Work out the finished part from the listing and answer in its coordinate system (mm). A direction names the side the tool comes from. Give positions to 0.01 mm unless a question says otherwise; leave off trailing zeros. Loops run counter-clockwise (first coordinate to the right, second up) from the corner with the lowest first, then second, coordinate; pieces in that order, holes last. Notation, with made-up numbers: (-3.75, 81) - (0.25, 81) arc R17 ccw to (0.25, 94) - close; hole circle Ø8 at (64, 7.5). An arc over 180 degrees is marked (long way). Use CSV: the item, a comma, the result in double quotes.
from build123d import *

# Parameters (mm, degrees)
BOSS_EXTRUDE1_DEPTH          = 54.00000000000001
CUT_EXTRUDE1_REACH           = 79.096
SKETCH4_W                    = 49.00000000000001
SKETCH4_H                    = 9.930000000000003
CUT_EXTRUDE2_DEPTH           = 9.930000000000001
CUT_EXTRUDE3_DEPTH           = 9.930000000000001
CUT_EXTRUDE4_REACH           = 79.096
CUT_EXTRUDE5_DEPTH           = 3.5
CUT_EXTRUDE6_DEPTH           = 3.5
CUT_EXTRUDE7_DEPTH           = 3.5
CUT_EXTRUDE8_DEPTH           = 3.5
DRAFT1_ANGLE                 = 0.01722183664478431
F_5_0_5_DIAMETER_HOLE1_D     = 5
F_5_0_5_DIAMETER_HOLE1_DEPTH = 29.6
F_5_0_5_DIAMETER_HOLE2_D     = 5
F_5_0_5_DIAMETER_HOLE2_DEPTH = 26.5
FILLET1_R                    = 2
FILLET2_R                    = 5
FILLET3_R                    = 0.4999999999999998
FILLET5_R                    = 2.9999999999999996
BOSS_EXTRUDE2_DEPTH          = 21
FILLET4_R                    = 0.9999999999999991


with BuildPart() as part:
    # Sketch1 → Boss-Extrude1 (new body)
    with BuildSketch(Plane(origin=(0, 0, 0), x_dir=(-1, 0, 0), z_dir=(0, 0, -1))):
        Polygon((-28.5, 28.5), (-28.5, -28.51414849795304), (28.5, -28.49701556553382), (28.5, 28.5), align=None)
    extrude(amount=-BOSS_EXTRUDE1_DEPTH)

    # Cut-Extrude1: up to this plane
    cut_extrude1_end = Plane(origin=(28.5, -28.51414849795304, 54.00000000000001), z_dir=(-0.0003005777481625158, -0.9999999548265077, 0))
    # Sketch3 → Cut-Extrude1 (cut, up to the surface)
    with BuildSketch(Plane(origin=(0, -18.57, 0), x_dir=(1, 0, 0), z_dir=(0, 1, 0)), mode=Mode.PRIVATE) as cut_extrude1_sk1:
        Polygon((28.499999999999996, -5.000000000000003), (18.57, -5.000000000000004), (18.570000000000004, -54), (28.499999999999996, -53.99999999999999), align=None)
    cut_extrude1_tool1 = split(extrude(cut_extrude1_sk1.sketch, amount=-CUT_EXTRUDE1_REACH, mode=Mode.PRIVATE), bisect_by=cut_extrude1_end, keep=Keep.BOTH, mode=Mode.PRIVATE)
    add(cut_extrude1_tool1.solids().sort_by_distance((23.535, -18.57, 29.5))[0], mode=Mode.SUBTRACT)

    # Sketch4 → Cut-Extrude2 (cut)
    with BuildSketch(Plane(origin=(28.5, 0, 0), x_dir=(0, 0, -1), z_dir=(1, 0, 0))):
        with Locations((-29.500000000000004, 23.535000000000004)):
            Rectangle(SKETCH4_W, SKETCH4_H)
    extrude(amount=-CUT_EXTRUDE2_DEPTH, mode=Mode.SUBTRACT)

    # Sketch5 → Cut-Extrude3 (cut)
    with BuildSketch(Plane(origin=(0, 28.5, 0), x_dir=(-1, 0, 0), z_dir=(0, 1, 0))):
        Polygon((18.570000000000004, 5.000000000000003), (28.499999999999996, 5.000000000000003), (28.5, 54), (18.57, 54), align=None)
    extrude(amount=-CUT_EXTRUDE3_DEPTH, mode=Mode.SUBTRACT)

    # Cut-Extrude4: up to this plane
    cut_extrude4_end = Plane(origin=(28.5, -28.51414849795304, 54.00000000000001), z_dir=(-0.0003005777481625158, -0.9999999548265077, 0))
    # Sketch7 → Cut-Extrude4 (cut, up to the surface)
    with BuildSketch(Plane(origin=(0, -18.57, 0), x_dir=(1, 0, 0), z_dir=(0, 1, 0)), mode=Mode.PRIVATE) as cut_extrude4_sk1:
        Polygon((-18.569999999999997, -5.000000000000004), (-28.499999999999996, -5.000000000000003), (-28.5, -54), (-18.569999999999997, -53.99999999999999), align=None)
    cut_extrude4_tool1 = split(extrude(cut_extrude4_sk1.sketch, amount=-CUT_EXTRUDE4_REACH, mode=Mode.PRIVATE), bisect_by=cut_extrude4_end, keep=Keep.BOTH, mode=Mode.PRIVATE)
    add(cut_extrude4_tool1.solids().sort_by_distance((-23.535, -18.57, 29.5))[0], mode=Mode.SUBTRACT)

    # Sketch8 → Cut-Extrude5 (cut)
    with BuildSketch(Plane(origin=(0, 0, 0), x_dir=(-1, 0, 0), z_dir=(0, 0, -1))):
        with BuildLine():
            Line((18.5710070868336, -28.5), (18.569999848669397, -25.148993064543653))
            ThreePointArc((18.569999848669397, -25.148993064543653), (15.21959273974545, -21.800000024754763), (11.870000005525402, -25.149807585039706))
            Line((11.870000005525402, -25.149807585039706), (11.869807463820973, -28.502014231583665))
            Line((11.869807463820973, -28.502014231583665), (18.5710070868336, -28.5))
        make_face()
    extrude(amount=-CUT_EXTRUDE5_DEPTH, mode=Mode.SUBTRACT)

    # Sketch9 → Cut-Extrude6 (cut)
    with BuildSketch(Plane(origin=(0, 0, 0), x_dir=(-1, 0, 0), z_dir=(0, 0, -1))):
        with BuildLine():
            Line((-18.57, 28.5), (-18.57, 25.15))
            ThreePointArc((-18.57, 25.15), (-15.22, 21.799999999999997), (-11.87, 25.15))
            Line((-11.87, 25.15), (-11.87, 28.5))
            Line((-11.87, 28.5), (-18.57, 28.5))
        make_face()
    extrude(amount=-CUT_EXTRUDE6_DEPTH, mode=Mode.SUBTRACT)

    # Sketch10 → Cut-Extrude7 (cut)
    with BuildSketch(Plane(origin=(0, 0, 0), x_dir=(-1, 0, 0), z_dir=(0, 0, -1))):
        with BuildLine():
            Line((-25.15, -11.870000000000003), (-28.5, -11.87))
            Line((-28.5, -11.87), (-28.5, -18.57))
            Line((-28.5, -18.57), (-25.15, -18.57))
            ThreePointArc((-25.15, -18.57), (-21.799999999999997, -15.22), (-25.15, -11.870000000000003))
        make_face()
    extrude(amount=-CUT_EXTRUDE7_DEPTH, mode=Mode.SUBTRACT)

    # Sketch11 → Cut-Extrude8 (cut)
    with BuildSketch(Plane(origin=(0, 0, 0), x_dir=(-1, 0, 0), z_dir=(0, 0, -1))):
        with BuildLine():
            Line((28.5, 18.57), (25.15, 18.57))
            ThreePointArc((25.15, 18.57), (21.799999999999997, 15.22), (25.15, 11.869999999999992))
            Line((25.15, 11.869999999999992), (28.5, 11.87))
            Line((28.5, 11.87), (28.5, 18.57))
        make_face()
    extrude(amount=-CUT_EXTRUDE8_DEPTH, mode=Mode.SUBTRACT)

    # Draft1
    draft1_faces = [part.faces().sort_by_distance(p)[0] for p in [
        (0.17151026292326854, -28.505633583914378, 26.11567870035269),
    ]]
    draft(draft1_faces, Plane(origin=(-18.5710070868336, -28.5, 3.5), x_dir=(0.00030057774815282144, 0.9999999548265077, 0), z_dir=(0.9999999548265077, -0.00030057774815282144, 0)), DRAFT1_ANGLE)

    # Sketch12 → Revolve1 (revolve)
    with BuildSketch(Plane(origin=(0, 0, 0), x_dir=(1, 0, 0), z_dir=(0, 1, 0))):
        Polygon((3.2500000000000004, 24.6), (0, 24.6), (0, 0), (19.05, 0), (19.05, 1.6), (3.2500000000000004, 1.6000000000000008), align=None)
    revolve(axis=Axis((0, 0, -24.6), (0, 0, 1)))

    # Ø5.0 (5) Diameter Hole1
    with Locations(Plane.XY.offset(5.000000000000008)):
        with Locations((23.57, -23.57), (23.57, 23.57), (-23.57, 23.57), (-23.57, -23.57)):
            Hole(F_5_0_5_DIAMETER_HOLE1_D / 2, depth=F_5_0_5_DIAMETER_HOLE1_DEPTH)

    # Ø5.0 (5) Diameter Hole2
    with Locations(Plane(origin=(0, 0, 3.5), x_dir=(-1, 0, 0), z_dir=(0, 0, -1))):
        with Locations((15.22, -25.15), (-25.15, -15.22), (-15.22, 25.15), (25.15, 15.22)):
            Hole(F_5_0_5_DIAMETER_HOLE2_D / 2, depth=F_5_0_5_DIAMETER_HOLE2_DEPTH)

    # Fillet1
    fillet1_edges = [part.edges().sort_by_distance(p)[0] for p in [
        (28.499999999999996, -18.57, 29.499999999999996),
        (18.570000000000004, -28.49999999999951, 29.50000000000001),
        (18.57, 28.5, 29.500000000000004),
        (28.5, 18.57, 29.5),
        (-28.499999999999996, 18.57, 29.500000000000004),
        (-18.57, 28.5, 29.5),
        (-28.499999999999996, -18.57, 29.500000000000004),
        (-18.57, -28.5, 29.500000000000007),
    ]]
    fillet(fillet1_edges, radius=FILLET1_R)

    # Fillet2
    fillet2_edges = [part.edges().sort_by_distance(p)[0] for p in [
        (18.57, -18.57, 29.5),
        (18.57, 18.57, 29.5),
        (-18.57, 18.57, 29.5),
        (-18.569999999999997, -18.57, 29.5),
    ]]
    fillet(fillet2_edges, radius=FILLET2_R)

    # Fillet3
    fillet3_edges = [part.edges().sort_by_distance(p)[0] for p in [
        (-3.2500000000000004, 4e-16, -24.6),
    ]]
    fillet(fillet3_edges, radius=FILLET3_R)

    # Fillet5
    fillet5_edges = [part.edges().sort_by_distance(p)[0] for p in [
        (28.5, -28.499999999999375, 2.5000000000000013),
        (28.5, 28.5, 2.5000000000000013),
        (-28.5, 28.5, 2.5000000000000013),
        (-28.5, -28.500000000000135, 2.5000000000000013),
    ]]
    fillet(fillet5_edges, radius=FILLET5_R)

    # Sketch17 → Boss-Extrude2 (add)
    with BuildSketch(Plane.XY.offset(54.00000000000001)):
        with BuildLine():
            Line((-16.570000000000007, 28.5), (16.569999999999983, 28.5))
            ThreePointArc((16.569999999999983, 28.5), (17.98421356237308, 27.914213562373096), (18.57, 26.500000000000004))
            Line((18.57, 26.500000000000004), (18.57, 23.57))
            ThreePointArc((18.57, 23.57), (20.034466094067263, 20.034466094067263), (23.57, 18.57))
            Line((23.57, 18.57), (26.499999999999996, 18.57))
            ThreePointArc((26.499999999999996, 18.57), (27.914213562373096, 17.984213562373093), (28.5, 16.569999999999993))
            Line((28.5, 16.569999999999993), (28.500000000000004, -16.569999999999997))
            ThreePointArc((28.500000000000004, -16.569999999999997), (27.9142135623731, -17.984213562373093), (26.500000000000004, -18.57))
            Line((26.500000000000004, -18.57), (23.569999999999986, -18.57))
            ThreePointArc((23.569999999999986, -18.57), (20.034466094067255, -20.034466094067263), (18.57, -23.57))
            Line((18.57, -23.57), (18.570000000000004, -26.499999999999538))
            ThreePointArc((18.570000000000004, -26.499999999999538), (17.98421356237311, -27.914213562372627), (16.57000000000003, -28.499999999999535))
            Line((16.57000000000003, -28.499999999999535), (-16.56999999999997, -28.49999999999997))
            ThreePointArc((-16.56999999999997, -28.49999999999997), (-17.98421356237307, -27.91421356237308), (-18.569999999999993, -26.49999999999999))
            Line((-18.569999999999993, -26.49999999999999), (-18.569999999999997, -23.57))
            ThreePointArc((-18.569999999999997, -23.57), (-20.034466094067266, -20.034466094067255), (-23.570000000000014, -18.57))
            Line((-23.570000000000014, -18.57), (-26.500000000000004, -18.57))
            ThreePointArc((-26.500000000000004, -18.57), (-27.9142135623731, -17.984213562373096), (-28.5, -16.57))
            Line((-28.5, -16.57), (-28.5, 16.57))
            ThreePointArc((-28.5, 16.57), (-27.914213562373096, 17.984213562373093), (-26.500000000000004, 18.57))
            Line((-26.500000000000004, 18.57), (-23.570000000000004, 18.57))
            ThreePointArc((-23.570000000000004, 18.57), (-20.034466094067266, 20.034466094067263), (-18.57, 23.57))
            Line((-18.57, 23.57), (-18.570000000000004, 26.500000000000004))
            ThreePointArc((-18.570000000000004, 26.500000000000004), (-17.984213562373103, 27.9142135623731), (-16.570000000000007, 28.5))
        make_face()
    extrude(amount=BOSS_EXTRUDE2_DEPTH)

    # Fillet4
    fillet4_edges = [part.edges().sort_by_distance(p)[0] for p in [
        (-17.984213562373103, 27.9142135623731, 75),
        (-18.57, 25.035000000000004, 75),
        (-20.034466094067266, 20.034466094067263, 75),
        (-25.035000000000004, 18.57, 75),
        (-27.914213562373096, 17.984213562373093, 75),
        (-28.5, 0, 75),
        (-27.9142135623731, -17.984213562373096, 75),
        (-25.03500000000001, -18.57, 75),
        (-20.034466094067263, -20.034466094067255, 75),
        (-18.569999999999993, -25.034999999999997, 75),
        (-17.98421356237307, -27.91421356237308, 75),
        (2.842e-14, -28.49999999999975, 75),
        (17.98421356237311, -27.914213562372627, 75),
        (18.57, -25.03499999999977, 75),
        (20.034466094067252, -20.034466094067263, 75),
        (25.034999999999997, -18.57, 75),
        (27.9142135623731, -17.984213562373093, 75),
        (28.5, 0, 75),
        (27.914213562373096, 17.984213562373093, 75),
        (25.034999999999997, 18.57, 75),
        (20.034466094067263, 20.034466094067263, 75),
        (18.57, 25.035000000000004, 75),
        (17.984213562373082, 27.914213562373096, 75),
        (-1.421e-14, 28.5, 75),
    ]]
    fillet(fillet4_edges, radius=FILLET4_R)


solid = part.part
Item 1: A cutting plane is placed at C-C on z = 10.5. Determine the outline of the cut face in (x, y).
Determined:
outline,"(-28.5, -16.57) arc R2 ccw to (-26.5, -18.57) - (-23.57, -18.57) arc R5 cw to (-18.57, -23.57) - (-18.57, -26.5) arc R2 ccw to (-16.57, -28.5) - (16.57, -28.5) arc R2 ccw to (18.57, -26.5) - (18.57, -23.57) arc R5 cw to (23.57, -18.57) - (26.5, -18.57) arc R2 ccw to (28.5, -16.57) - (28.5, 16.57) arc R2 ccw to (26.5, 18.57) - (23.57, 18.57) arc R5 cw to (18.57, 23.57) - (18.57, 26.5) arc R2 ccw to (16.57, 28.5) - (-16.57, 28.5) arc R2 ccw to (-18.57, 26.5) - (-18.57, 23.57) arc R5 cw to (-23.57, 18.57) - (-26.5, 18.57) arc R2 ccw to (-28.5, 16.57) - close; hole circle Ø5 at (-25.15, 15.22); hole circle Ø5 at (-15.22, -25.15); hole circle Ø5 at (15.22, 25.15); hole circle Ø5 at (25.15, -15.22)"
Item 2: The mould has two halves that part along X. Classify faces 6 (the flat face through (27.4, -16.7, 3.5)), 7 (the cylindrical face through (15.3, 21.8, 1.7)), 8 (the cylindrical face through (-27.9, 18, 39)), 9 (the cylindrical face through (-15.3, -21.8, 1.7)): pulls with the +X half, pulls with the -X half, needs draft (parallel to the pull), parting line crosses it, or undercut.
Determined:
face 6,"needs draft"
face 7,"undercut"
face 8,"pulls with the -X half"
face 9,"undercut"
Item 3: A cutting plane is placed at D-D on y = 6. Determine the outline of the cut face in (x, z).
Determined:
outline,"(-28.5, 0) - (-18.08, 0) - (-18.08, -1.6) - (18.08, -1.6) - (18.08, 0) - (28.5, 0) - (28.5, 74) arc R1 ccw to (27.5, 75) - (-27.5, 75) arc R1 ccw to (-28.5, 74) - close"
Item 4: A cutting plane is placed at B-B on x = 0. Determine the outline of the cut face in (y, z), and give its area (3 significant figures).
Determined:
outline,"(-28.5, 0) - (-19.05, 0) - (-19.05, -1.6) - (-3.25, -1.6) - (-3.25, -24.1) arc R0.5 ccw to (-2.75, -24.6) - (2.75, -24.6) arc R0.5 ccw to (3.25, -24.1) - (3.25, -1.6) - (19.05, -1.6) - (19.05, 0) - (28.5, 0) - (28.5, 74) arc R1 ccw to (27.5, 75) - (-27.5, 75) arc R1 ccw to (-28.5, 74) - close"
area,"4,480 mm²"
Item 5: Find the intervals of material crossed by line 1 (X direction, y = 23, z = 2); line 2 (Y direction, x = -25.15, z = 22); line 3 (Y direction, x = -15.22, z = 16), in increasing order.
Determined:
line 1,"x = -28.5 to -26, -21.14 to 12.65, 17.79 to 21.14, 26 to 28.5"
line 2,"y = -18.57 to 12.72, 17.72 to 18.57"
line 3,"y = -28.5 to -27.65, -22.65 to 28.5"
Item 6: For faces 1 (the flat face through (23.9, -26.4, 5)), 2 (the cylindrical face through (-0.705, -3.173, -13.008)), 3 (the flat face through (-18.57, -25, 39)), 4 (the cylindrical face through (20, 20.07, 39.02)), 5 (the cylindrical face through (21.8, -15.3, 1.7)), determine the directions among +Z, -Z, +X, -X, +Y, -Y from which every point of the face is accessible in a straight line to the end or side of a thin tool.
Determined:
face 1,"+Z, +X, -Y"
face 2,"-Z"
face 3,"+Z, -X, -Y"
face 4,"+Z, +X, +Y"
face 5,"-Z, +X"
Item 7: Given P1, Ø5, axis at y = -15, z = -1.5, coming from the -X side; P2, Ø6, axis at x = -23.57, y = -23.57, coming from the +Z side; P3, Ø7.5, axis at x = -25, y = 15.5, coming from the -Z side; P4, Ø2.5, axis at x = -25, z = 43.5, coming from the +Y side, each flat-ended and moving along its own axis, determine where each tip first touches the part or whether it passes through.
Determined:
P1,"stops at x = -28.5"
P2,"stops at z = 5"
P3,"stops at z = 0"
P4,"stops at y = 18.57"
Item 8: A cutting plane is placed at A-A on z = 66. Determine the outline of the cut face in (x, y).
Determined:
outline,"(-28.5, -16.57) arc R2 ccw to (-26.5, -18.57) - (-23.57, -18.57) arc R5 cw to (-18.57, -23.57) - (-18.57, -26.5) arc R2 ccw to (-16.57, -28.5) - (16.57, -28.5) arc R2 ccw to (18.57, -26.5) - (18.57, -23.57) arc R5 cw to (23.57, -18.57) - (26.5, -18.57) arc R2 ccw to (28.5, -16.57) - (28.5, 16.57) arc R2 ccw to (26.5, 18.57) - (23.57, 18.57) arc R5 cw to (18.57, 23.57) - (18.57, 26.5) arc R2 ccw to (16.57, 28.5) - (-16.57, 28.5) arc R2 ccw to (-18.57, 26.5) - (-18.57, 23.57) arc R5 cw to (-23.57, 18.57) - (-26.5, 18.57) arc R2 ccw to (-28.5, 16.57) - close"
